from build123d import *

# Parameters (mm, degrees)
F0_W     = 30
F0_H     = 50
F1_DEPTH = 25
F2_W     = 30
F2_H     = 25
F3_DEPTH = 25
F4_R     = 15
F5_DEPTH = 25


with BuildPart() as f1:
    # F0 (on Top) → F1 (new body)
    with BuildSketch(Plane.XY):
        with Locations((-15, -25)):
            Rectangle(F0_W, F0_H)
    extrude(amount=F1_DEPTH)

    # F2 (on face) → F3 (join)
    with BuildSketch(Plane(origin=(0, 0, 0), x_dir=(-1, 0, 0), z_dir=(0, 1, 0))):
        with BuildLine():
            Line((-10, 100), (-10, 0))
            Line((-10, 0), (0, 0))
            Line((0, 0), (0, 25))
            Line((0, 25), (30, 25))
            Line((30, 25), (30, 0))
            Line((30, 0), (40, 0))
            Line((40, 0), (40, 100))
            ThreePointArc((40, 100), (15, 125), (-10, 100))
        make_face()
        with Locations((15, 12.5)):
            Rectangle(F2_W, F2_H)
    extrude(amount=-F3_DEPTH)

    # F4 (on face) → F5 (cut)
    with BuildSketch(Plane.XZ.offset(25)):
        with Locations((-15, 100)):
            Circle(F4_R)
    extrude(amount=-F5_DEPTH, mode=Mode.SUBTRACT)


solid = f1.part
Can you work these out from the model? Positions are in its coordinate system, mm. A direction names the side the tool comes from. Round coordinates to 2 decimals unless told otherwise and drop trailing zeros. Order: outer loops, then holes, each group sorted by start corner. A loop starts at its lowest first (then second) coordinate and runs counter-clockwise, first axis right, second up. Notation, with made-up numbers: M 11,32.25 L 54,32.25 A33 cw 54,67.25 Z; hole C 64,47.25 d8. An arc over 180 degrees is marked long. Use a Markdown table: item, result.
1) Imagine slicing it at A-A (x = -15). List the corners of the cut face in (y, z) for me, then the cut area to 3 significant figures.
Geometry says:
| item | result |
|---|---|
| outline | M -50,0 L 0,0 L 0,85 L -25,85 L -25,25 L -50,25 Z; M -25,115 L 0,115 L 0,125 L -25,125 Z |
| area | 3,000 mm² |
2) If I drill on line 1 along Z through (x, y) = (-15, -17); line 2 along Y through (x, z) = (-17, 29); line 3 along X through (y, z) = (-9.5, 89.5), over which ranges is the centre line in solid material (lowest first)?
Geometry says:
| item | result |
|---|---|
| line 1 | z = 0 to 85, 115 to 125 |
| line 2 | y = -25 to 0 |
| line 3 | x = -40 to -25.71, -4.29 to 10 |
3) Imagine slicing it at C-C (z = 113). List the corners of the cut face in (x, y) for me, then the cut area to 3 significant figures.
Geometry says:
| item | result |
|---|---|
| outline | M -36.35,-25 L -22.48,-25 L -22.48,0 L -36.35,0 Z; M -7.52,-25 L 6.35,-25 L 6.35,0 L -7.52,0 Z |
| area | 694 mm² |
4) On a 3-axis mill with a long thin cutter (end or side, diameter ignored), from which of +Z, -Z, +X, -X, +Y, -Y can I reach the whole of each face in a straight line? I mean faces 1 (the face through (-15, -37, 25)), 2 (the face through (-15, -50, 12)), 3 (the face through (0, -38, 12)). Say none if no direction works.
Geometry says:
| item | result |
|---|---|
| face 1 | +Z, +X, -X, -Y |
| face 2 | +Z, -Z, +X, -X, -Y |
| face 3 | +Z, -Z, +X, -Y |
5) I'm going to push flat-ended pins straight in: P1, Ø18, axis at x = -15, z = 100, coming from the -Y side; P2, Ø3, axis at x = -15, y = -26, coming from the -Z side; P3, Ø12.5, axis at y = -41.5, z = 7, coming from the -X side; P4, Ø7.5, axis at x = -19.5, y = -33.5, coming from the +Z side. Where does each tip first touch, or does it pass through?
Geometry says:
| item | result |
|---|---|
| P1 | passes through |
| P2 | stops at z = 0 |
| P3 | stops at x = -30 |
| P4 | stops at z = 25 |
6) Imagine slicing it at B-B (y = -20). List the corners of the cut face in (x, z) for me, then the cut area to 3 significant figures.
Geometry says:
| item | result |
|---|---|
| outline | M -40,0 L 10,0 L 10,100 A25 ccw -40,100 Z; hole C -15,100 d30 |
| area | 5,270 mm² |
7) If we mould it in two halves opening along X, with no side actions, what happens to faces 4 (the face through (-18.252, -12.675, 85.357)), 5 (the face through (-15.55, -12.325, 124.994)), 6 (the face through (-30, -38, 12)), 7 (the face through (10, -12, 51))? For each: +X half, -X half, draft (parallel to the pull), parting line (faces both ways), or undercut.
Geometry says:
| item | result |
|---|---|
| face 4 | undercut |
| face 5 | parting line |
| face 6 | -X half |
| face 7 | +X half |
8) Imagine slicing it at D-D (z = 88.5). List the corners of the cut face in (x, y) for me, then the cut area to 3 significant figures.
Geometry says:
| item | result |
|---|---|
| outline | M -40,-25 L -24.63,-25 L -24.63,0 L -40,0 Z; M -5.37,-25 L 10,-25 L 10,0 L -5.37,0 Z |
| area | 768 mm² |
